Can you work these out from the model? Positions are in its coordinate system, mm. Coordinates: 2 decimals unless noted, no trailing zeros. Order: outer loops, then holes, each group sorted by start corner. A loop starts at its lowest first (then second) coordinate and runs counter-clockwise, first axis right, second up. Notation, with made-up numbers: (-12, 87) - (8, 87) arc R29 ccw to (8, 119) - close; hole circle Ø5 at (0.5, 87). An arc over 180 degrees is marked (long way). Return JSON: item names as keys, results as strings. Group by question number.
1) If I drill on line 1 along X through (y, z) = (-12.5, 2.5); line 2 along Y through (x, z) = (-11.5, 17), over which ranges is the centre line in solid material (lowest first)?
2) Imagine slicing it at D-D (z = 24.5). Write out the boundary of the cut face in (x, y), and give its area (3 significant figures).
3) Imagine slicing it at C-C (x = 4.5). Write out the boundary of the cut face in (y, z).
4) Imagine slicing it at A-A (x = 9). Write out the boundary of the cut face in (y, z), and give its area (3 significant figures).
5) For pin 1 Ø10 at (x, z) = (-8.5, 19) entering from +Y; pin 2 Ø1.5 at (y, z) = (1, 35.5) entering from +X; pin 3 Ø1 at (y, z) = (1, 25) entering from -X, each with a flat end and sliding along its axis, tell me the tip position at first contact or that it passes through.
6) Imagine slicing it at B-B (y = -11.5). Write out the boundary of the cut face in (x, z), and give its area (3 significant figures).
7) If we mould it in two halves opening along Y, with no side actions, what happens to faces 1 (the face through (-13.163, 11.994, 20.213)), 2 (the face through (0, 0, 41)), 3 (the face through (-4.336, -19.524, 20.213))? For each: pulls with the +Y half, pulls with the -Y half, needs draft (parallel to the pull), parting line crosses it, or undercut.
```python
from build123d import *

# Parameters (mm, degrees)
SKETCH2_R           = 20
BOSS_EXTRUDE1_DEPTH = 35
SKETCH5_R           = 20
BOSS_EXTRUDE4_DEPTH = 6
SKETCH6_R           = 5
CUT_EXTRUDE1_DEPTH  = 50.809637622
CIRPATTERN2_COUNT   = 4


with BuildPart() as part:
    # Sketch2 → Boss-Extrude1 (new body)
    with BuildSketch(Plane.XY):
        Circle(SKETCH2_R)
    extrude(amount=BOSS_EXTRUDE1_DEPTH)

    # Sketch5 → Boss-Extrude4 (add)
    with BuildSketch(Plane.XY.offset(35)):
        Circle(SKETCH5_R)
    extrude(amount=BOSS_EXTRUDE4_DEPTH)

    # Sketch6 → Cut-Extrude1 (cut, through all)
    with BuildSketch(Plane(origin=(0, 0, 0), x_dir=(-1, 0, 0), z_dir=(0, 0, -1))):
        with Locations((-11.343432643, 8.205274881)):
            Circle(SKETCH6_R)
    cut_extrude1 = extrude(amount=-CUT_EXTRUDE1_DEPTH, mode=Mode.SUBTRACT)

    # CirPattern2: Cut-Extrude1 ×4 about axis
    cirpattern2_axis = Axis((0, 0, 0), (0, 0, 1))
    for i in range(1, CIRPATTERN2_COUNT):
        add(cut_extrude1.rotate(cirpattern2_axis, i * 360 / CIRPATTERN2_COUNT), mode=Mode.SUBTRACT)


solid = part.part
```
Calculated:
{
 "1": {"line 1": "-15.61 to -13.9, -8.78 to 3.34, 13.07 to 15.61", "line 2": "-16.36 to -13.2, -3.21 to 7.58, 15.1 to 16.36"},
 "2": {"outline": "circle Ø40 at (0, 0); hole circle Ø10 at (-11.34, -8.21); hole circle Ø10 at (-8.21, 11.34); hole circle Ø10 at (8.21, -11.34); hole circle Ø10 at (11.34, 8.21)", "area": "942 mm2"},
 "3": {"outline": "(-19.49, 0) - (-14.7, 0) - (-14.7, 41) - (-19.49, 41) - close; (-7.99, 0) - (19.49, 0) - (19.49, 41) - (-7.99, 41) - close"},
 "4": {"outline": "(-17.86, 0) - (-16.28, 0) - (-16.28, 41) - (-17.86, 41) - close; (-6.41, 0) - (3.79, 0) - (3.79, 41) - (-6.41, 41) - close; (12.62, 0) - (17.86, 0) - (17.86, 41) - (12.62, 41) - close", "area": "698 mm2"},
 "5": {"pin 1": "y = 19.69", "pin 2": "x = 20", "pin 3": "x = -19.99"},
 "6": {"outline": "(-16.36, 0) - (-15.1, 0) - (-15.1, 41) - (-16.36, 41) - close; (-7.58, 0) - (3.21, 0) - (3.21, 41) - (-7.58, 41) - close; (13.2, 0) - (16.36, 0) - (16.36, 41) - (13.2, 41) - close", "area": "624 mm2"},
 "7": {"face 1": "undercut", "face 2": "needs draft", "face 3": "parting line crosses it"}
}
